The drawing under review shows one solid part. Ordinate dimensions are in mm from its lowest x, y, z. A direction names the side the tool comes from. Coordinates: 2 decimals unless noted, no trailing zeros.
1) For P1, Ø4.5, axis at y = 9.525, z = 9.525, coming from the -X side; P2, Ø6.5, axis at y = 71.5, z = 9, coming from the -X side, all flat-tipped, find the tip position at first contact; note any pin that passes through.
2) Mouldability with a two-part tool opening along X and no side actions: class the marked faces 3, 4 and 5 as released by +X, released by -X, zero draft, split by the parting line, or undercut.
3) Machinability: for the marked faces 1 and 2, which of the approach directions +Z, -Z, +X, -X, +Y, -Y give a long, thin tool a straight path to every point of the face, cutting with its end or side? Answer none if there is none.
4) For line 1 (Z direction, x = 5.5, y = 26); line 2 (Z direction, x = 18.25, y = 15); line 3 (Z direction, x = 1, y = 58.5), list the stretches that pass through material, from the lowest coordinate up.
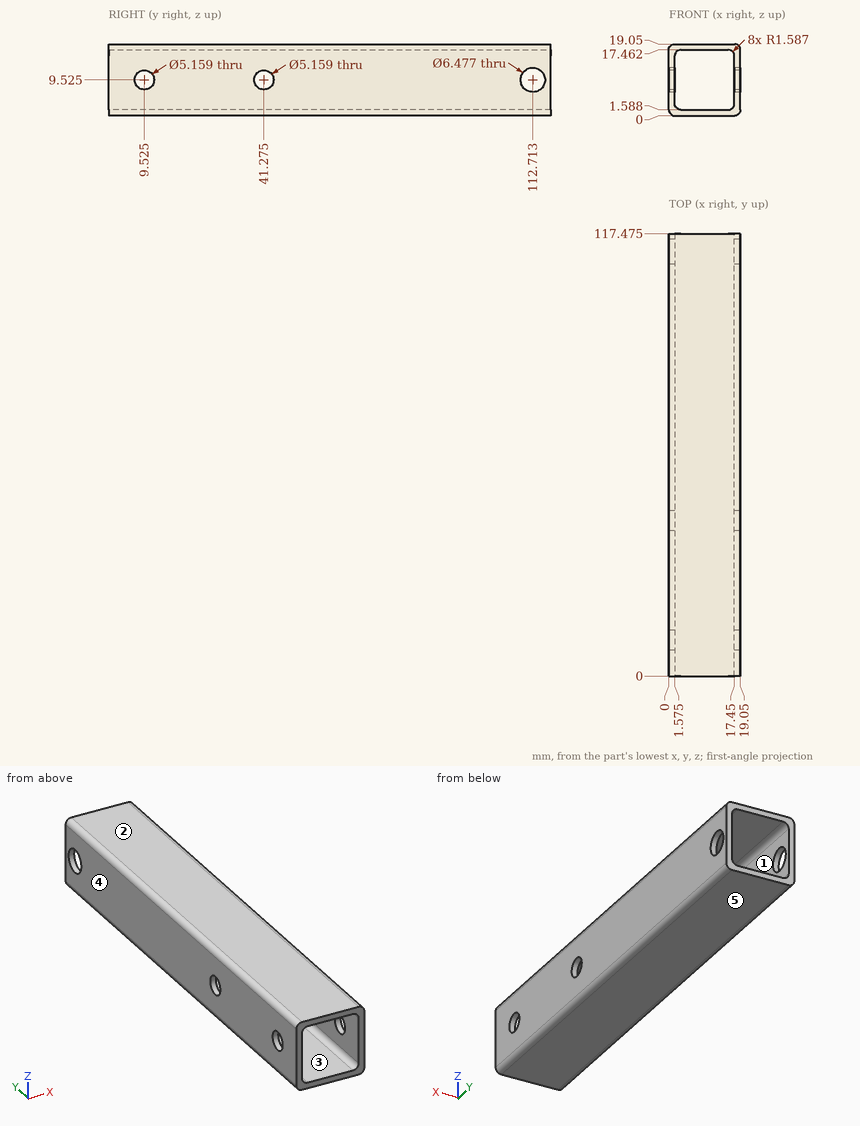
Geometry results:
1. P1: passes through
1. P2: stops at x = 0
2. face 3: undercut
2. face 4: released by -X
2. face 5: zero draft
3. face 1: +Y, -Y
3. face 2: +Z, +X, -X, +Y, -Y
4. line 1: z = 0 to 1.59, 17.46 to 19.05
4. line 2: z = 0.21 to 18.84
4. line 3: z = 0.11 to 18.94
